```python
from build123d import *

# Parameters (mm, degrees)
BOSS_EXTRUDE1_DEPTH = 4
SKETCH2_R           = 1.25
CUT_EXTRUDE1_DEPTH  = 4
SKETCH6_R           = 2.5
SKETCH6_W           = 30.2
SKETCH6_H           = 66.1
CUT_EXTRUDE5_DEPTH  = 4
CUT_EXTRUDE6_DEPTH  = 4


with BuildPart() as part:
    # Sketch1 → Boss-Extrude1 (new body)
    with BuildSketch(Plane(origin=(0, 0, 0), x_dir=(1, 0, 0), z_dir=(0, 1, 0))):
        with BuildLine():
            Line((-17.5, 0), (-17.5, 118))
            Line((-17.5, 118), (17.5, 118))
            Line((17.5, 118), (17.5, 0))
            ThreePointArc((17.5, 0), (0, -17.5), (-17.5, 0))
        make_face()
    extrude(amount=BOSS_EXTRUDE1_DEPTH)

    # Sketch2 → Cut-Extrude1 (cut)
    with BuildSketch(Plane(origin=(0, 4, 0), x_dir=(1, 0, 0), z_dir=(0, 1, 0))):
        with Locations((-8.75, 0)):
            Circle(SKETCH2_R)
        with Locations((8.75, 0)):
            Circle(SKETCH2_R)
    extrude(amount=-CUT_EXTRUDE1_DEPTH, mode=Mode.SUBTRACT)

    # Sketch6 → Cut-Extrude5 (cut)
    with BuildSketch(Plane(origin=(0, 4, 0), x_dir=(1, 0, 0), z_dir=(0, 1, 0))):
        with Locations((-8.9, 37.7)):
            Circle(SKETCH6_R)
        with Locations((8.9, 37.7)):
            Circle(SKETCH6_R)
        with Locations((8.9, 112.2)):
            Circle(SKETCH6_R)
        with Locations((-8.9, 112.2)):
            Circle(SKETCH6_R)
        with Locations((0, 74.95)):
            Rectangle(SKETCH6_W, SKETCH6_H)
    extrude(amount=-CUT_EXTRUDE5_DEPTH, mode=Mode.SUBTRACT)

    # Sketch7 → Cut-Extrude6 (cut)
    with BuildSketch(Plane(origin=(0, 4, 0), x_dir=(1, 0, 0), z_dir=(0, 1, 0))):
        Polygon((0, 41.9), (-2.5, 41.9), (-2.5, 33.4), (2.5, 33.4), (2.5, 41.9), align=None)
        Polygon((2.5, 108), (0, 108), (-2.5, 108), (-2.5, 116.5), (2.5, 116.5), align=None)
    extrude(amount=-CUT_EXTRUDE6_DEPTH, mode=Mode.SUBTRACT)


solid = part.part
```
Can you work these out from the model? Positions are in its coordinate system, mm. A direction names the side the tool comes from. Round coordinates to 2 decimals unless told otherwise and drop trailing zeros. Loops run counter-clockwise (first coordinate to the right, second up) from the corner with the lowest first, then second, coordinate; pieces in that order, holes last. Notation, with made-up numbers: M -29.75,12.25 L -5.75,12.25 A18 cw -5.75,38.25 Z; hole C -18,-21 d2. An arc over 180 degrees is marked long. Answer in a Markdown table with one row per item.
1. If we section it at D-D, the plane x = 8.75: Please give me the cut outline in (y, z).
Established:
| item | result |
|---|---|
| outline | M 0,-118 L 4,-118 L 4,-114.7 L 0,-114.7 Z; M 0,-109.7 L 4,-109.7 L 4,-108 L 0,-108 Z; M 0,-41.9 L 4,-41.9 L 4,-40.2 L 0,-40.2 Z; M 0,-35.2 L 4,-35.2 L 4,-1.25 L 0,-1.25 Z; M 0,1.25 L 4,1.25 L 4,15.16 L 0,15.16 Z |
2. Please list where these lines run through material, in increasing order: line 1 (X direction, y = 2.4, z = -37.7); line 2 (X direction, y = 3.3, z = -65); line 3 (Z direction, x = -8.75, y = 2.3). Write a range as from..to.
Established:
| item | result |
|---|---|
| line 1 | -17.5..-11.4, -6.4..-2.5, 2.5..6.4, 11.4..17.5 |
| line 2 | -17.5..-15.1, 15.1..17.5 |
| line 3 | -118..-114.7, -109.7..-108, -41.9..-40.2, -35.2..-1.25, 1.25..15.16 |
3. I'm going to push flat-ended pins straight in: pin 1 Ø3 at (x, z) = (-8.9, -37.7) entering from +Y; pin 2 Ø2 at (x, y) = (-10.5, 3) entering from +Z. Where does each tip first touch, or does it pass through?
Established:
| item | result |
|---|---|
| pin 1 | through |
| pin 2 | z = 14.7 |
4. If we section it at C-C, the plane y = 1.45: Please give me the cut outline in (x, z).
Established:
| item | result |
|---|---|
| outline | M -17.5,-118 L 17.5,-118 L 17.5,0 A17.5 ccw -17.5,0 Z; hole M -15.1,-108 L -2.5,-108 L -2.5,-116.5 L 2.5,-116.5 L 2.5,-108 L 15.1,-108 L 15.1,-41.9 L 2.5,-41.9 L 2.5,-33.4 L -2.5,-33.4 L -2.5,-41.9 L -15.1,-41.9 Z; hole C -8.9,-112.2 d5; hole C -8.9,-37.7 d5; hole C -8.75,0 d2.5; hole C 8.9,-112.2 d5; hole C 8.9,-37.7 d5; hole C 8.75,0 d2.5 |
5. If we section it at B-B, the plane z = -102.5: Please give me the cut outline in (x, y), plus the area to 3 significant figures.
Established:
| item | result |
|---|---|
| outline | M -17.5,0 L -15.1,0 L -15.1,4 L -17.5,4 Z; M 15.1,0 L 17.5,0 L 17.5,4 L 15.1,4 Z |
| area | 19.2 mm² |
6. Thinking about a two-plate mould opening in Z: for faces 3 (the face through (0.385, 1.972, 17.496)), 4 (the face through (15.1, 2, -74)), 5 (the face through (-17.5, 2, -58)), which applies, pulls with the +Z half, pulls with the -Z half, needs draft (parallel to the pull), parting line crosses it, or undercut?
Established:
| item | result |
|---|---|
| face 3 | pulls with the +Z half |
| face 4 | undercut |
| face 5 | needs draft |
7. If we section it at A-A, the plane z = -37.7: Please give me the cut outline in (x, y), plus the area to 3 significant figures.
Established:
| item | result |
|---|---|
| outline | M -17.5,0 L -11.4,0 L -11.4,4 L -17.5,4 Z; M -6.4,0 L -2.5,0 L -2.5,4 L -6.4,4 Z; M 2.5,0 L 6.4,0 L 6.4,4 L 2.5,4 Z; M 11.4,0 L 17.5,0 L 17.5,4 L 11.4,4 Z |
| area | 80.0 mm² |
8. On a 3-axis mill with a long thin cutter (end or side, diameter ignored), from which of +Z, -Z, +X, -X, +Y, -Y can I reach the whole of each face in a straight line? I mean faces 1 (the face through (-9, 2, -41.9)), 2 (the face through (4, 0, -36)). Say none if no direction works.
Established:
| item | result |
|---|---|
| face 1 | +Y, -Y |
| face 2 | +Z, -Z, +X, -X, -Y |
